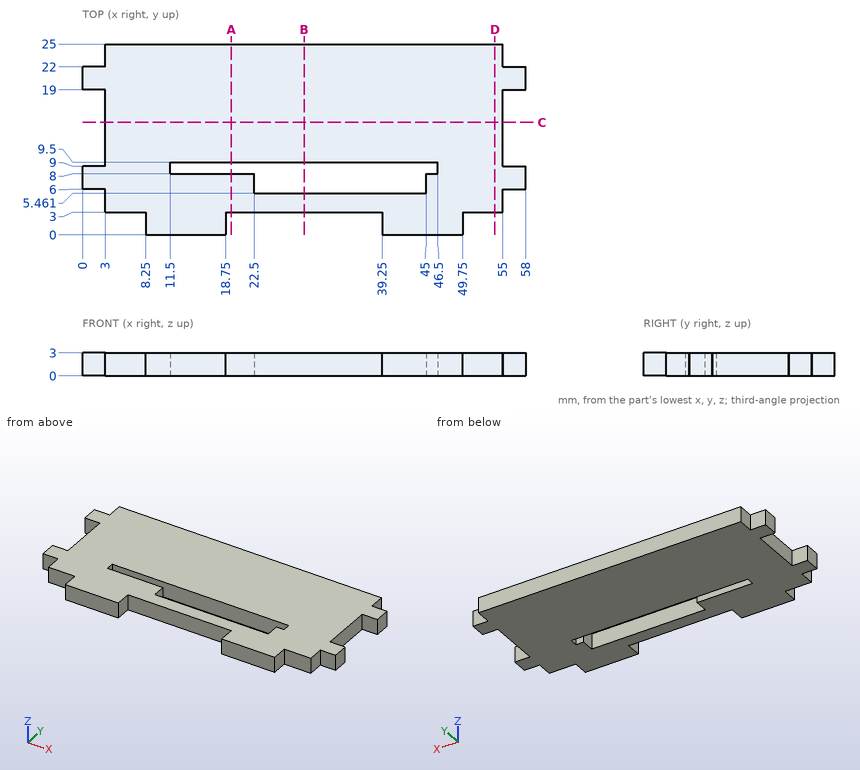
The drawing under review shows one solid part. Ordinate dimensions are in mm from its lowest x, y, z. Give positions to 0.01 mm unless a question says otherwise; leave off trailing zeros. Write each loop counter-clockwise with the first axis right and the second up, starting at its lowest first coordinate (ties: lowest second). Pieces come first, ordered by that corner, then holes. Notation, with made-up numbers: M 54.25,67 L 100.25,67 A15 ccw 100.25,79 Z; hole C 36,-16.5 d3. An arc over 180 degrees is marked long. Write each question's results on one line, items separated by ' | '. Start each with the question number.
1. We need section B-B (x = 29). Write out the cut boundary in (y, z).
2. We need section C-C (y = 14.75). Write out the cut boundary in (x, z), and give its area (3 significant figures).
3. Insertion check: pin 1 Ø0.9 at (y, z) = (23, 1.5) entering from +X; pin 2 Ø0.9 at (x, z) = (57, 2) entering from +Y; pin 3 Ø1.5 at (x, z) = (7, 1.5) entering from -Y. Each pin has a flat end and moves straight along its axis. Give the tip position at first contact, or say it passes through.
4. For probe 1 along Y at (x, z) = (27, 2.75); probe 2 along X at (y, z) = (8.75, 2.25); probe 3 along Y at (x, z) = (51, 2.5), list the stretches that pass through material, from the lowest coordinate up. Write a range as [from, to].
5. We need section A-A (x = 19.5). Write out the cut boundary in (y, z), and give its area (3 significant figures).
6. We need section D-D (x = 54). Write out the cut boundary in (y, z).
Results found:
1) outline: M 3,0 L 5.46,0 L 5.46,3 L 3,3 Z; M 9.5,0 L 25,0 L 25,3 L 9.5,3 Z
2) outline: M 3,0 L 55,0 L 55,3 L 3,3 Z | area: 156 mm^2
3) pin 1: stops at x = 55 | pin 2: stops at y = 22 | pin 3: stops at y = 3
4) probe 1: y = [3, 5.46], [9.5, 25] | probe 2: x = [0, 11.5], [46.5, 58] | probe 3: y = [3, 25]
5) outline: M 3,0 L 8,0 L 8,3 L 3,3 Z; M 9.5,0 L 25,0 L 25,3 L 9.5,3 Z | area: 61.5 mm^2
6) outline: M 3,0 L 25,0 L 25,3 L 3,3 Z
